Autodesk Inventor part; units mm, degrees
ref_plane "YZ Plane" through (0, 0, 0) normal (1, 0, 0) x (0, 1, 0)
ref_plane "XZ Plane" through (0, 0, 0) normal (0, 1, 0) x (-1, 0, 0)
ref_plane "XY Plane" through (0, 0, 0) normal (0, 0, 1) x (1, 0, 0)
sketch "Sketch1" plane through (0, 0, 0) normal (1, 0, 0) x (0, 1, 0)
  line L0 (0, 0) -> (250, 0)
  line L1 (250, 0) -> (250, -25.4)
  dimension "d0" = 25.4
  dimension "d1" = 250
contour flange "Contour Flange1" sketch "Sketch1" thickness 3.175 bend radius 3.175 width 350 along (1, 0, 0) mid plane no both sides no wall seen from (0, 125, 0) lies toward (0, 0, -1) curves L0 L1
bend "Bend1"
corner "Corner1"
sketch "Sketch2" plane through (0, 0, 0) normal (0, 0, 1) x (1, 0, 0)
  line L0 (350, 0) -> (350, 243.65)
  line L1 (0, 0) -> (0, 243.65)
  line L2 (0, 243.65) -> (350, 243.65)
  line L3 (0, 0) -> (0, 243.65)
  line L4 (350, 0) -> (0, 0)
  line L5 (350, 243.65) -> (350, 0)
  arc A0 (269.2821, 77.9424) -> (167.772, 75.6113) centre (237.5885, -753.3037) ccw
  arc A1 (167.772, 75.6113) -> (0, 43.8953) centre (237.5885, -753.3037) ccw
  arc A2 (350, 70.916) -> (269.2821, 77.9424) centre (237.5885, -753.3037) ccw
  point P0 (0, 61.7144)
  point P1 (350, 0)
  point P2 (350, 70.916)
  point P3 (0, 43.8953)
extrude "Cut1" cut sketch "Sketch2" against normal blind 3.175 contours L4 L1 A1 A0 A2 L0
sketch "Sketch7" plane through (0, 243.65, 0) normal (0, 0, 1) x (1, 0, 0)
  line L0 (350, 0) -> (350, -172.734) construction
  line L1 (0, 0) -> (350, 0) construction
  line L2 (0, -199.7547) -> (0, 0) construction
  line L3 (350, -202.0252) -> (265.0055, 6.35)
  line L4 (0, 6.35) -> (350, 6.35) construction
  line L5 (350, -202.0252) -> (350, 6.35)
  line L6 (350, 6.35) -> (265.0055, 6.35)
  arc A0 (350, -172.734) -> (0, -199.7547) centre (237.5885, -996.9537) ccw
  point P0 (0, -243.65)
  point P1 (346.825, 6.35)
  dimension "d56" = 22.19
extrude "Cut4" cut sketch "Sketch7" along normal through all both and the other way through all
equation "\"d14\" = Thickness"
equation "\"d57\" = Thickness"
equation "\"d2\" = Thickness"
equation "\"d3\" = BendReliefWidth"
equation "\"d4\" = BendReliefDepth"
equation "\"d5\" = MinimumRemnant"
equation "\"d6\" = TransitionRadius"
equation "\"d8\" = BendRadius"
equation "\"d10\" = CornerReliefSize"
equation "\"d11\" = GapSize"
equation "\"d12\" = JacobiRadiusSize"
equation "\"BendRadius\" = Thickness"
equation "\"BendReliefWidth\" = Thickness"
equation "\"BendReliefDepth\" = 0.5 * Thickness"
equation "\"CornerReliefSize\" = 4 * Thickness"
equation "\"MinimumRemnant\" = 2 * Thickness"
equation "\"TransitionRadius\" = BendRadius"
equation "\"JacobiRadiusSize\" = BendRadius"
equation "\"GapSize\" = Thickness"
properties part number "SIDE_INTAKE_LEXAN" material "Polycarbonate, PC 1000, Clear"
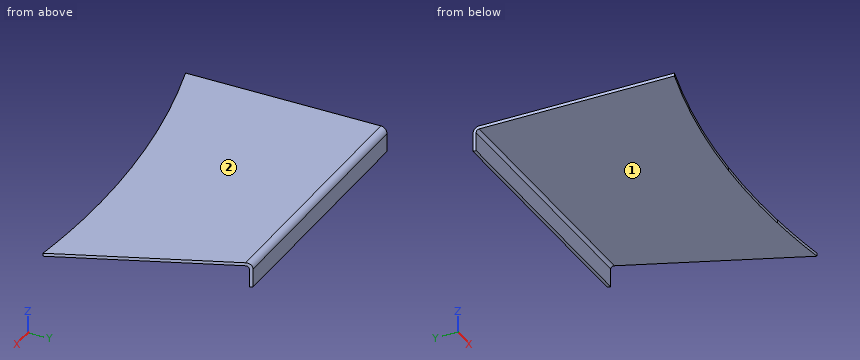
Design review of the part built by this model. Coordinates are the model's own, in mm. Face numbers are marked on the shaded views. A direction names the side the tool comes from. Round coordinates to 2 decimals unless told otherwise and drop trailing zeros. Order: outer loops, then holes, each group sorted by start corner. A loop starts at its lowest first (then second) coordinate and runs counter-clockwise, first axis right, second up. Notation, with made-up numbers: (33, 21.5) - (52, 21.5) arc R24 cw to (52, 40.5) - close; hole circle Ø5 at (52.25, 61.5). An arc over 180 degrees is marked (long way). Return JSON: item names as keys, results as strings.
Q1. Consider section D-D on x = 202.5. Write out the cut boundary in (y, z) (3 decimals), plus the area to 3 significant figures.
Computed values:
{"outline": "(77.806, -3.175) - (243.65, -3.175) arc R3.175 cw to (246.825, -6.35) - (246.825, -25.4) - (250, -25.4) - (250, -6.35) arc R6.35 ccw to (243.65, 0) - (77.806, 0) - close", "area": "611 mm2"}
Q2. Consider section A-A on x = 50.5. Write out the cut boundary in (y, z) (3 decimals).
Computed values:
{"outline": "(57.235, -3.175) - (243.65, -3.175) arc R3.175 cw to (246.825, -6.35) - (246.825, -25.4) - (250, -25.4) - (250, -6.35) arc R6.35 ccw to (243.65, 0) - (57.235, 0) - close"}
Q3. Consider section B-B on z = -20.5. Write out the cut boundary in (x, y) (1 decimal).
Computed values:
{"outline": "(0, 246.8) - (266.3, 246.8) - (265, 250) - (0, 250) - close"}
Q4. Consider section C-C on y = 167. Write out the cut boundary in (x, z) (1 decimal), plus the area to 3 significant figures.
Computed values:
{"outline": "(0, -3.2) - (298.9, -3.2) - (298.9, 0) - (0, 0) - close", "area": "949 mm2"}
Q5. For pin 1 Ø3 at (x, z) = (232, -15.5) entering from -Y (3 decimals), flat-tipped, find the tip position at first contact; note if it passes through.
Computed values:
{"pin 1": "stops at y = 246.825"}
Q6. Wall thickness on L1, parallel to Y at x = 74.5, z = -13.25 (3 decimals); L2, parallel to Z at x = 57, y = 221 (3 decimals); L3, parallel to X at y = 120, z = -2: over which ranges is each line inside the solid? List them lowest first. Write a range as [from, to].
Computed values:
{"L1": "y = [246.825, 250]", "L2": "z = [-3.175, 0]", "L3": "x = [0, 318.03]"}
Q7. Machinability: for the marked faces 1 and 2, which of the approach directions +Z, -Z, +X, -X, +Y, -Y give a long, thin tool a straight path to every point of the face, cutting with its end or side? Answer none if there is none.
Computed values:
{"face 1": "-Z, +X, -X, -Y", "face 2": "+Z, +X, -X, +Y, -Y"}
